For this review, take the finished solid that the model builds, in its own axes (mm). Round coordinates to 2 decimals unless told otherwise and drop trailing zeros. Loops run counter-clockwise (first coordinate to the right, second up) from the corner with the lowest first, then second, coordinate; pieces in that order, holes last.
1. Consider section A-A on x = 35. State the section outline as (y, z) points, then the cut area to 3 significant figures.
2. Consider section D-D on z = -16. State the section outline as (x, y) points.
3. Consider section C-C on x = 18. State the section outline as (y, z) points, then the cut area to 3 significant figures.
4. Consider section B-B on z = -52. State the section outline as (x, y) points.
5. To check wall thickness, follow line 1 along Y through (x, z) = (2, -22); line 2 along X through (y, z) = (24, -93). State the ranges of each line that lie inside material, in increasing order.
6. Draft analysis for pull direction Z (two halves, no side actions). For faces 1 (the flat face through (54, 18, 3)), 2 (the cylindrical face through (1.52, 12.95, -83.43)), 3 (the flat face through (1, 17, -97)), 4 (the cylindrical face through (23.5, 12.57, 1.52)), state which applies: released by +Z, released by -Z, zero draft, split by the parting line, or undercut.
7. Clearance check with flat-ended pins moving along their axes: pin 1 Ø4 at (x, y) = (75, 22.5) entering from -Z; pin 2 Ø3.5 at (y, z) = (32.5, -12) entering from +X; pin 3 Ø5 at (x, y) = (15, 32.5) entering from -Z; pin 4 Ø5 at (y, z) = (11, -82) entering from -X. State where each tip first meets the part, or that it passes through.
from build123d import *

# Parameters (mm, degrees)
ESQUISSE1_W             = 100
ESQUISSE1_H             = 35
BOSS_EXTRU_1_DEPTH      = 3
ESQUISSE2_R             = 1.5
ENL_V_MAT_EXTRU_1_DEPTH = 3
ESQUISSE5_W             = 100
ESQUISSE5_H             = 35
BOSS_EXTRU_2_DEPTH      = 3
ESQUISSE6_R             = 1.5
ENL_V_MAT_EXTRU_2_DEPTH = 3
CONG_1_SIZE             = 10
CONG_2_R                = 1


with BuildPart() as part:
    # Esquisse1 → Boss.-Extru.1 (new body)
    with BuildSketch(Plane.XY):
        with Locations((50, 17.5)):
            Rectangle(ESQUISSE1_W, ESQUISSE1_H)
    extrude(amount=BOSS_EXTRU_1_DEPTH)

    # Esquisse2 → Enlèv. mat.-Extru.1 (cut)
    with BuildSketch(Plane.XY.offset(3)):
        with Locations((95, 32.5)):
            Circle(ESQUISSE2_R)
        with Locations((85, 32.5)):
            Circle(ESQUISSE2_R)
        with Locations((75, 32.5)):
            Circle(ESQUISSE2_R)
        with Locations((65, 32.5)):
            Circle(ESQUISSE2_R)
        with Locations((55, 32.5)):
            Circle(ESQUISSE2_R)
        with Locations((45, 32.5)):
            Circle(ESQUISSE2_R)
        with Locations((35, 32.5)):
            Circle(ESQUISSE2_R)
        with Locations((25, 32.5)):
            Circle(ESQUISSE2_R)
        with Locations((15, 32.5)):
            Circle(ESQUISSE2_R)
        with Locations((85, 22.5)):
            Circle(ESQUISSE2_R)
        with Locations((75, 22.5)):
            Circle(ESQUISSE2_R)
        with Locations((65, 22.5)):
            Circle(ESQUISSE2_R)
        with Locations((55, 22.5)):
            Circle(ESQUISSE2_R)
        with Locations((45, 22.5)):
            Circle(ESQUISSE2_R)
        with Locations((35, 22.5)):
            Circle(ESQUISSE2_R)
        with Locations((25, 22.5)):
            Circle(ESQUISSE2_R)
        with Locations((15, 22.5)):
            Circle(ESQUISSE2_R)
        with Locations((85, 12.5)):
            Circle(ESQUISSE2_R)
        with Locations((75, 12.5)):
            Circle(ESQUISSE2_R)
        with Locations((65, 12.5)):
            Circle(ESQUISSE2_R)
        with Locations((55, 12.5)):
            Circle(ESQUISSE2_R)
        with Locations((45, 12.5)):
            Circle(ESQUISSE2_R)
        with Locations((35, 12.5)):
            Circle(ESQUISSE2_R)
        with Locations((25, 12.5)):
            Circle(ESQUISSE2_R)
        with Locations((15, 12.5)):
            Circle(ESQUISSE2_R)
        with Locations((85, 2.5)):
            Circle(ESQUISSE2_R)
        with Locations((75, 2.5)):
            Circle(ESQUISSE2_R)
        with Locations((65, 2.5)):
            Circle(ESQUISSE2_R)
        with Locations((55, 2.5)):
            Circle(ESQUISSE2_R)
        with Locations((45, 2.5)):
            Circle(ESQUISSE2_R)
        with Locations((35, 2.5)):
            Circle(ESQUISSE2_R)
        with Locations((25, 2.5)):
            Circle(ESQUISSE2_R)
        with Locations((15, 2.5)):
            Circle(ESQUISSE2_R)
        with Locations((95, 22.5)):
            Circle(ESQUISSE2_R)
        with Locations((95, 12.5)):
            Circle(ESQUISSE2_R)
        with Locations((95, 2.5)):
            Circle(ESQUISSE2_R)
    extrude(amount=-ENL_V_MAT_EXTRU_1_DEPTH, mode=Mode.SUBTRACT)

    # Esquisse5 → Boss.-Extru.2 (add)
    with BuildSketch(Plane.ZY):
        with Locations((-47, 17.5)):
            Rectangle(ESQUISSE5_W, ESQUISSE5_H)
    extrude(amount=-BOSS_EXTRU_2_DEPTH)

    # Esquisse6 → Enlèv. mat.-Extru.2 (cut)
    with BuildSketch(Plane(origin=(3, 0, 0), x_dir=(0, 0, -1), z_dir=(1, 0, 0))):
        with Locations((92, 32.5)):
            Circle(ESQUISSE6_R)
        with Locations((82, 32.5)):
            Circle(ESQUISSE6_R)
        with Locations((72, 32.5)):
            Circle(ESQUISSE6_R)
        with Locations((62, 32.5)):
            Circle(ESQUISSE6_R)
        with Locations((52, 32.5)):
            Circle(ESQUISSE6_R)
        with Locations((42, 32.5)):
            Circle(ESQUISSE6_R)
        with Locations((32, 32.5)):
            Circle(ESQUISSE6_R)
        with Locations((22, 32.5)):
            Circle(ESQUISSE6_R)
        with Locations((12, 32.5)):
            Circle(ESQUISSE6_R)
        with Locations((82, 22.5)):
            Circle(ESQUISSE6_R)
        with Locations((72, 22.5)):
            Circle(ESQUISSE6_R)
        with Locations((62, 22.5)):
            Circle(ESQUISSE6_R)
        with Locations((52, 22.5)):
            Circle(ESQUISSE6_R)
        with Locations((42, 22.5)):
            Circle(ESQUISSE6_R)
        with Locations((32, 22.5)):
            Circle(ESQUISSE6_R)
        with Locations((22, 22.5)):
            Circle(ESQUISSE6_R)
        with Locations((12, 22.5)):
            Circle(ESQUISSE6_R)
        with Locations((82, 12.5)):
            Circle(ESQUISSE6_R)
        with Locations((72, 12.5)):
            Circle(ESQUISSE6_R)
        with Locations((62, 12.5)):
            Circle(ESQUISSE6_R)
        with Locations((52, 12.5)):
            Circle(ESQUISSE6_R)
        with Locations((42, 12.5)):
            Circle(ESQUISSE6_R)
        with Locations((32, 12.5)):
            Circle(ESQUISSE6_R)
        with Locations((22, 12.5)):
            Circle(ESQUISSE6_R)
        with Locations((12, 12.5)):
            Circle(ESQUISSE6_R)
        with Locations((82, 2.5)):
            Circle(ESQUISSE6_R)
        with Locations((72, 2.5)):
            Circle(ESQUISSE6_R)
        with Locations((62, 2.5)):
            Circle(ESQUISSE6_R)
        with Locations((52, 2.5)):
            Circle(ESQUISSE6_R)
        with Locations((42, 2.5)):
            Circle(ESQUISSE6_R)
        with Locations((32, 2.5)):
            Circle(ESQUISSE6_R)
        with Locations((22, 2.5)):
            Circle(ESQUISSE6_R)
        with Locations((12, 2.5)):
            Circle(ESQUISSE6_R)
        with Locations((92, 22.5)):
            Circle(ESQUISSE6_R)
        with Locations((92, 12.5)):
            Circle(ESQUISSE6_R)
        with Locations((92, 2.5)):
            Circle(ESQUISSE6_R)
    extrude(amount=-ENL_V_MAT_EXTRU_2_DEPTH, mode=Mode.SUBTRACT)

    # Congé1
    # a fillet whose section is not a circle: 10 mm, written as the material it adds along each edge
    with BuildSketch(Plane(origin=(3, 35, 0), x_dir=(1, 0, 0), z_dir=(0, -1, 0))) as cong_1_piece_1:
        with BuildLine():
            Bezier((CONG_1_SIZE, 0), (0, 0), (0, -CONG_1_SIZE), weights=[1, 0.333333333, 1])
            Line((0, -CONG_1_SIZE), (0, 0))
            Line((0, 0), (CONG_1_SIZE, 0))
        make_face()
    extrude(amount=35)
    # a fillet whose section is not a circle: 10 mm, written as the material it takes off along each edge
    with BuildSketch(Plane(origin=(0, 60, 3), x_dir=(1, 0, 0), z_dir=(0, -1, 0))) as cong_1_2_piece_1:
        with BuildLine():
            Bezier((CONG_1_SIZE, 0), (0, 0), (0, -CONG_1_SIZE), weights=[1, 0.333333333, 1])
            Line((0, -CONG_1_SIZE), (0, 0))
            Line((0, 0), (CONG_1_SIZE, 0))
        make_face()
    extrude(amount=85, mode=Mode.SUBTRACT)

    # Congé2
    cong_2_edges = [part.edges().sort_by_distance(p)[0] for p in [
        (100, 35, 1.5),
        (100, 0, 1.5),
        (1.5, 0, -97),
        (1.5, 35, -97),
    ]]
    fillet(cong_2_edges, radius=CONG_2_R)


solid = part.part
Resolved:
1. outline: (0, 0) - (1, 0) - (1, 3) - (0, 3) - close; (4, 0) - (11, 0) - (11, 3) - (4, 3) - close; (14, 0) - (21, 0) - (21, 3) - (14, 3) - close; (24, 0) - (31, 0) - (31, 3) - (24, 3) - close; (34, 0) - (35, 0) - (35, 3) - (34, 3) - close
1. area: 69.0 mm2
2. outline: (0, 0) - (3, 0) - (3, 35) - (0, 35) - close
3. outline: (0, 0) - (35, 0) - (35, 3) - (0, 3) - close
3. area: 105 mm2
4. outline: (0, 0) - (3, 0) - (3, 1) - (0, 1) - close; (0, 4) - (3, 4) - (3, 11) - (0, 11) - close; (0, 14) - (3, 14) - (3, 21) - (0, 21) - close; (0, 24) - (3, 24) - (3, 31) - (0, 31) - close; (0, 34) - (3, 34) - (3, 35) - (0, 35) - close
5. line 1: y = 0 to 1, 4 to 11, 14 to 21, 24 to 31, 34 to 35
5. line 2: x = 0 to 3
6. face 1: released by +Z
6. face 2: undercut
6. face 3: released by -Z
6. face 4: zero draft
7. pin 1: stops at z = 0
7. pin 2: stops at x = 3
7. pin 3: stops at z = -0.05
7. pin 4: stops at x = 0
